from build123d import *

# Parameters (mm, degrees)
F0_R     = 1.5875
F1_DEPTH = 3.175


with BuildPart() as f1:
    # F0 (on Right) → F1 (new body)
    with BuildSketch(Plane.YZ):
        with BuildLine():
            ThreePointArc((-38.625983, 6.35), (-36.766111, 1.859872), (-32.275983, 0))
            Line((-32.275983, 0), (-32.032519, 0))
            Line((-32.032519, 0), (-11.197744, 0))
            Line((-11.197744, 0), (-11.197744, -3.175))
            Line((-11.197744, -3.175), (-0.780357, -3.175))
            Line((-0.780357, -3.175), (-0.780357, 0))
            Line((-0.780357, 0), (20.054419, 0))
            Line((20.054419, 0), (20.054419, -3.175))
            Line((20.054419, -3.175), (30.471806, -3.175))
            Line((30.471806, -3.175), (30.471806, 0))
            Line((30.471806, 0), (51.306581, 0))
            ThreePointArc((51.306581, 0), (56.690855, 2.983682), (57.015299, 9.130835))
            Line((57.015299, 9.130835), (53.459318, 16.430835))
            ThreePointArc((53.459318, 16.430835), (51.116919, 19.034273), (47.7506, 20))
            Line((47.7506, 20), (-28.720002, 20))
            Line((-28.720002, 20), (-32.275983, 20))
            ThreePointArc((-32.275983, 20), (-36.766111, 18.140128), (-38.625983, 13.65))
            Line((-38.625983, 13.65), (-38.625983, 6.35))
        make_face()
        with BuildLine():
            ThreePointArc((-25.020661, 7.661057), (-36.428301, 10), (-25.020661, 12.338943))
            ThreePointArc((-25.020661, 12.338943), (-22.153501, 10), (-25.020661, 7.661057))
        make_face(mode=Mode.SUBTRACT)
        with Locations((-5.484701, 10)):
            Circle(F0_R, mode=Mode.SUBTRACT)
        with Locations((4.515299, 10)):
            Circle(F0_R, mode=Mode.SUBTRACT)
        with Locations((39.515299, 10)):
            Circle(F0_R, mode=Mode.SUBTRACT)
    extrude(amount=F1_DEPTH)


solid = f1.part
Geometry: final body of the model. Coordinates: model frame, mm. A direction names the side the tool comes from. Give positions to 0.01 mm unless a question says otherwise; leave off trailing zeros. Loops run counter-clockwise (first coordinate to the right, second up) from the corner with the lowest first, then second, coordinate; pieces in that order, holes last. Notation, with made-up numbers: M -7.75,-27 L -1.75,-27 A15 cw -1.75,-2 Z; hole C 69.25,75 d9. An arc over 180 degrees is marked long. Put each result on its own line as item: value. Start each with the question number.
1) Cut plane B-B (z = 14.75). Output: boundary loops of the cut face in (x, y) (3 decimals).
2) Access query for faces 1 (the flat face through (2, 20.054, -2)), 2 (the cylindrical face through (1.565, -36.716, 18.189)), 3 (the flat face through (2, 30.472, -2)). Directions: +Z, -Z, +X, -X, +Y, -Y. A direction counts if a zero-diameter tool reaches every point of the face in a straight line with its end or side. Return the directions, or none.
3) Cut plane D-D (z = 10). Output: boundary loops of the cut face in (x, y) (1 decimal), then the cut area to 3 significant figures.
4) Cut plane A-A (y = -5). Output: boundary loops of the cut face in (x, z) (3 decimals).
5) Ray query, line 1 along Y through (x, z) = (1, 10.5); line 2 along Z through (x, y) = (1.5, 0); line 3 along Y through (x, z) = (0.4, 10.75). Return the intervals inside material, ascending.
6) Cut plane C-C (x = 1.9). Give the number of separate pieces and of enclosed holes in the cut face, then the cut area to 3 significant figures.
7) Contact query for flat-ended pins moving along their axis: pin 1 (7.5 mm diameter, centred on y = -24.54, z = 10, fed in from -X); pin 2 (1 mm diameter, centred on x = 2, z = 2, fed in from -Y); pin 3 (1 mm diameter, centred on x = 2.5, z = -1.5, fed in from +Y); pin 4 (1 mm diameter, centred on x = 2, y = 37, fed in from -Z). Output: stop coordinate, or through.
8) Pull-direction query (Y, two-part tool) for faces 4 (the flat face through (1.57, 55.26, 12.73)), 5 (the flat face through (2, -22, 0)), 6 (the flat face through (2, -0.78, -2)), 7 (the flat face through (2, -11.198, -2)); classes: pulls with the +Y half, pulls with the -Y half, needs draft (parallel to the pull), parting line crosses it, or undercut.
Verdict:
1. outline: M 0,-38.53 L 3.175,-38.53 L 3.175,-34.057 L 0,-34.057 Z; M 0,-26.912 L 3.175,-26.912 L 3.175,54.278 L 0,54.278 Z
2. face 1: -Z, +X, -X
2. face 2: +Z, +X, -X, -Y
2. face 3: -Z, +X, -X, +Y
3. outline: M 0,-38.6 L 3.2,-38.6 L 3.2,-36.4 L 0,-36.4 Z; M 0,-22.2 L 3.2,-22.2 L 3.2,-7.1 L 0,-7.1 Z; M 0,-3.9 L 3.2,-3.9 L 3.2,2.9 L 0,2.9 Z; M 0,6.1 L 3.2,6.1 L 3.2,37.9 L 0,37.9 Z; M 0,41.1 L 3.2,41.1 L 3.2,56.6 L 0,56.6 Z
3. area: 227 mm2
4. outline: M 0,-3.175 L 3.175,-3.175 L 3.175,8.488 L 0,8.488 Z; M 0,11.512 L 3.175,11.512 L 3.175,20 L 0,20 Z
5. line 1: -38.63 to -36.41, -22.21 to -6.99, -3.98 to 3.01, 6.02 to 38.01, 41.02 to 56.35
5. line 2: 0 to 20
5. line 3: -38.63 to -36.38, -22.27 to -6.88, -4.09 to 3.12, 5.91 to 38.12, 40.91 to 56.23
6. separate pieces: 1
6. enclosed holes: 4
6. area: 1,780 mm2
7. pin 1: x = 0
7. pin 2: y = -37.33
7. pin 3: y = 30.47
7. pin 4: z = 0
8. face 4: pulls with the +Y half
8. face 5: needs draft
8. face 6: undercut
8. face 7: pulls with the -Y half
